```python
from build123d import *

# Parameters (mm, degrees)
RESSALTO_EXTRUS_O1_DEPTH = 30
ESBO_O2_R                = 1.6
CORTE_EXTRUS_O1_DEPTH    = 30


with BuildPart() as part:
    # Esboço1 → Ressalto-extrusão1 (new body)
    with BuildSketch(Plane.XY):
        with BuildLine():
            Line((0, 55), (0, 0))
            Line((0, 0), (7.886751346, 0))
            Line((7.886751346, 0), (23.330127019, 26.748711306))
            Line((23.330127019, 26.748711306), (21.598076211, 27.748711306))
            Line((21.598076211, 27.748711306), (7.598076211, 3.5))
            ThreePointArc((7.598076211, 3.5), (4.223542865, 2.102222521), (2, 5))
            Line((2, 5), (2, 55))
            Line((2, 55), (0, 55))
        make_face()
    extrude(amount=RESSALTO_EXTRUS_O1_DEPTH)

    # Esboço2 → Corte-extrusão1 (cut)
    with BuildSketch(Plane(origin=(4.183012702, -2.415063509, 0), x_dir=(0.5, 0.866025404, 0), z_dir=(-0.866025404, 0.5, 0))):
        with Locations((31.830127019, -27)):
            Circle(ESBO_O2_R)
        with Locations((7.830127019, -3)):
            Circle(ESBO_O2_R)
    extrude(amount=-CORTE_EXTRUS_O1_DEPTH, mode=Mode.SUBTRACT)


solid = part.part
```
Design review of the part built by this model. Coordinates are the model's own, in mm. A direction names the side the tool comes from. Round coordinates to 2 decimals unless told otherwise and drop trailing zeros. Write each loop counter-clockwise with the first axis right and the second up, starting at its lowest first coordinate (ties: lowest second). Pieces come first, ordered by that corner, then holes. Notation, with made-up numbers: (58, 11.25) -> (114, 11.25) arc R23 ccw to (114, 19.25) -> close; hole circle Ø4 at (13, 68). An arc over 180 degrees is marked (long way). Write item = value, one per line. Start each with the question number.
1) Tool access review of faces 5 (the face through (15.5, 13.19, 14.79)), 6 (the face through (2, 30, 15)): name each direction out of +Z, -Z, +X, -X, +Y, -Y from which nothing blocks a thin tool from reaching the whole face with its end or side.
2) Wall thickness on probe 1 along X at (y, z) = (44.5, 18); probe 2 along Z at (x, y) = (21.25, 25); probe 3 along X at (y, z) = (21, 18.75): over which ranges is each line inside the solid? List them lowest first. Write a range as from..to.
3) Take a section at A-A, the plane z = 8.5. State the section outline as (x, y) points.
4) Take a section at D-D, the plane x = 4.75. State the section outline as (y, z) points.
5) Clearance check with flat-ended pins moving along their axes: pin 1 (9 mm diameter, centred on y = 38, z = 17, fed in from +X); pin 2 (1.5 mm diameter, centred on x = 15.5, y = 9.5, fed in from -Z). State where each tip first meets the part, or that it passes through.
6) Mouldability with a two-part tool opening along Y and no side actions: class faces 1 (the face through (9.32, 4.51, 4.42)), 2 (the face through (1, 19, 30)), 3 (the face through (4.277, 2.088, 14.79)), 4 (the face through (20.848, 24.477, 25.414)) as +Y half, -Y half, draft (parallel to the pull), parting line (faces both ways), or undercut.
7) Take a section at B-B, the plane y = 15.5. State the section outline as (x, z) points.
8) Take a section at C-C, the plane y = 48. State the section outline as (x, z) points.
Results list:
q1.face_5 = +Z, -Z, +X, -Y
q1.face_6 = +Z, -Z, +Y
q2.probe_1 = 0..2
q2.probe_2 = 0..25.46, 28.54..30
q2.probe_3 = 0..2, 17.7..20.01
q3.outline = (0, 0) -> (7.89, 0) -> (23.33, 26.75) -> (21.6, 27.75) -> (7.6, 3.5) arc R3 cw to (2, 5) -> (2, 55) -> (0, 55) -> close
q4.outline = (0, 0) -> (2.01, 0) -> (2.01, 30) -> (0, 30) -> close
q5.pin_1 = 2
q5.pin_2 = through
q6.face_1 = undercut
q6.face_2 = draft
q6.face_3 = +Y half
q6.face_4 = undercut
q7.outline = (0, 0) -> (2, 0) -> (2, 30) -> (0, 30) -> close; (14.53, 0) -> (16.84, 0) -> (16.84, 30) -> (14.53, 30) -> close
q8.outline = (0, 0) -> (2, 0) -> (2, 30) -> (0, 30) -> close
